Read the model definition and answer for the solid it produces. Units are mm, in the model's axes. Round coordinates to 2 decimals unless told otherwise and drop trailing zeros. Order: outer loops, then holes, each group sorted by start corner. A loop starts at its lowest first (then second) coordinate and runs counter-clockwise, first axis right, second up. Notation, with made-up numbers: (47, -16) -> (79, -16) arc R22 cw to (79, 2) -> close; hole circle Ø9 at (25, -12.5). An arc over 180 degrees is marked (long way). Use a Markdown table: item, result. Add a question column.
1. Section D-D, the plane y = -11.5 is taken. Give the vertices of the cut face in (x, z), then the cut area to 3 significant figures.
2. The mould has two halves that part along Y. Classify faces 1 (the face through (-1, 0, 2.5)), 2 (the face through (49.506, 0.264, 1.268)): +Y half, -Y half, draft (parallel to the pull), parting line (faces both ways), or undercut.
3. Section C-C, the plane y = -21 is taken. Give the vertices of the cut face in (x, z).
4. Section B-B, the plane z = 1.05 is taken. Give the vertices of the cut face in (x, y).
5. Consider L1, parallel to Y at x = 55.5, z = 1.2; L2, parallel to Y at x = 36.5, z = 2.05; L3, parallel to Y at x = 13, z = 2.4. Determine where each line is inside the solid, lowest interval first. Write a range as [from, to].
6. Given pin 1 (14 mm diameter, centred on x = 55.5, y = 0, fed in from -Z), flat-ended and moving along its own axis, determine where the tip first touches the part or whether it passes through.
7. Section A-A, the plane x = 55.5 is taken. Give the vertices of the cut face in (y, z).
```python
from build123d import *

# Parameters (mm, degrees)
F0_W        = 194
F0_H        = 64.6
F1_DEPTH    = 2
F2_W        = 184
F2_H        = 54.6
F3_DEPTH    = 0.5
F4_R        = 6
F5_DEPTH    = 25
F6_T1_DEPTH = 16.5427907903
F6_T3_DEPTH = 2.4643962848


# Not quite as in the source:
# - a fillet or chamfer that OpenCascade refuses, or shapes differently, is made with other operations: its cross-section is extruded or revolved along the edge and cut away or added


with BuildPart() as f1:
    # F0 (on Top) → F1 (new body)
    with BuildSketch(Plane.XY):
        Rectangle(F0_W, F0_H)
        Polygon((98, 0), (97, 32.3), (97, -32.3), align=None)
        Polygon((-97, -32.3), (-97, 32.3), (-98, 0), align=None)
    extrude(amount=F1_DEPTH)

    # F2 (on face) → F3 (join)
    with BuildSketch(Plane.XY.offset(2)):
        Rectangle(F2_W, F2_H)
    extrude(amount=F3_DEPTH)

    # F4 (on face) → F5 (cut)
    with BuildSketch(Plane.XY.offset(2.5)):
        with Locations((36.5, 0)):
            Circle(F4_R)
        with Locations((55.5, 0)):
            Circle(F4_R)
    extrude(amount=-F5_DEPTH, mode=Mode.SUBTRACT)

    # F6: fillet of radius 3 on 6 edges, made by hand

    # F6_s2 → F6_t1 (cut)
    with BuildSketch(Plane.XY.offset(-7.2713953952)):
        with BuildLine():
            ThreePointArc((97.0900051153, -29.3928347763), (96.1796822102, -31.4538923289), (94.0914418419, -32.3))
            Line((94.0914418419, -32.3), (97, -32.3))
            Line((97, -32.3), (97.0900051153, -29.3928347763))
        make_face()
        with BuildLine():
            ThreePointArc((94.0914418419, 32.3), (96.1796822102, 31.4538923289), (97.0900051153, 29.3928347763))
            Line((97.0900051153, 29.3928347763), (97, 32.3))
            Line((97, 32.3), (94.0914418419, 32.3))
        make_face()
        with BuildLine():
            ThreePointArc((-94.0914418419, 32.3), (-96.1796822102, 31.4538923289), (-97.0900051153, 29.3928347763))
            Line((-97.0900051153, 29.3928347763), (-97, 32.3))
            Line((-97, 32.3), (-94.0914418419, 32.3))
        make_face()
        with BuildLine():
            ThreePointArc((-97.0900051153, -29.3928347763), (-96.1796822102, -31.4538923289), (-94.0914418419, -32.3))
            Line((-94.0914418419, -32.3), (-97, -32.3))
            Line((-97, -32.3), (-97.0900051153, -29.3928347763))
        make_face()
    extrude(amount=F6_T1_DEPTH, mode=Mode.SUBTRACT)

    # F6_s4 → F6_t3 (cut)
    with BuildSketch(Plane.XY.offset(-0.2321981424)):
        with BuildLine():
            ThreePointArc((-97.9971258583, 0.0928347763), (-97.998562585, 0), (-97.9971258583, -0.0928347763))
            Line((-97.9971258583, -0.0928347763), (-98, 0))
            Line((-98, 0), (-97.9971258583, 0.0928347763))
        make_face()
        with BuildLine():
            ThreePointArc((97.9971258583, 0.0928347763), (97.998562585, 0), (97.9971258583, -0.0928347763))
            Line((97.9971258583, -0.0928347763), (98, 0))
            Line((98, 0), (97.9971258583, 0.0928347763))
        make_face()
    extrude(amount=F6_T3_DEPTH, mode=Mode.SUBTRACT)


solid = f1.part
```
Verdict:
| question | item | result |
|---|---|---|
| 1 | outline | (-97.64, 0) -> (97.64, 0) -> (97.64, 2) -> (92, 2) -> (92, 2.5) -> (-92, 2.5) -> (-92, 2) -> (-97.64, 2) -> close |
| 1 | area | 483 mm2 |
| 2 | face 1 | draft |
| 2 | face 2 | undercut |
| 3 | outline | (-97.35, 0) -> (97.35, 0) -> (97.35, 2) -> (92, 2) -> (92, 2.5) -> (-92, 2.5) -> (-92, 2) -> (-97.35, 2) -> close |
| 4 | outline | (-98, -0.09) -> (-97.09, -29.39) arc R3 ccw to (-94.09, -32.3) -> (94.09, -32.3) arc R3 ccw to (97.09, -29.39) -> (98, -0.09) arc R3 ccw to (98, 0.09) -> (97.09, 29.39) arc R3 ccw to (94.09, 32.3) -> (-94.09, 32.3) arc R3 ccw to (-97.09, 29.39) -> (-98, 0.09) arc R3 ccw to start; hole circle Ø12 at (36.5, 0); hole circle Ø12 at (55.5, 0) |
| 5 | L1 | y = [-32.3, -6], [6, 32.3] |
| 5 | L2 | y = [-27.3, -6], [6, 27.3] |
| 5 | L3 | y = [-27.3, 27.3] |
| 6 | pin 1 | stops at z = 0 |
| 7 | outline | (-32.3, 0) -> (-6, 0) -> (-6, 2.5) -> (-27.3, 2.5) -> (-27.3, 2) -> (-32.3, 2) -> close; (6, 0) -> (32.3, 0) -> (32.3, 2) -> (27.3, 2) -> (27.3, 2.5) -> (6, 2.5) -> close |
